from build123d import *

# Parameters (mm, degrees)
SKETCH_1_W          = 35
SKETCH_1_H          = 3
EXTRUDE_1_DEPTH     = 25
EXTRUDE_1_2_DEPTH   = 25
SKETCH_2_W          = 35
SKETCH_2_H          = 9.3
EXTRUDE_2_DEPTH     = 70
SKETCH_3_R          = 1.5
CUT_EXTRUDE_1_DEPTH = 10


with BuildPart() as part:
    # Sketch 1 → Extrude 1 (new body)
    with BuildSketch(Plane.XY):
        with Locations((17.5, 1.5)):
            Rectangle(SKETCH_1_W, SKETCH_1_H)
    extrude(amount=EXTRUDE_1_DEPTH)



with BuildPart() as body_2:
    # Sketch 1 → Extrude 1 2 (new body)
    with BuildSketch(Plane.XY):
        with Locations((17.5, -4.8)):
            Rectangle(SKETCH_1_W, SKETCH_1_H)
    extrude(amount=EXTRUDE_1_2_DEPTH)


with BuildPart() as part_1:
    add(part.part)

    add(body_2.part)  # Extrude 2 merges body 2
    # Sketch 2 → Extrude 2 (add)
    with BuildSketch(Plane(origin=(0, 0, 0), x_dir=(-1, 0, 0), z_dir=(0, 0, -1))):
        with Locations((-17.5, -1.65)):
            Rectangle(SKETCH_2_W, SKETCH_2_H)
    extrude(amount=EXTRUDE_2_DEPTH)

    # Sketch 3 → Cut-Extrude 1 (cut)
    with BuildSketch(Plane(origin=(0, 3, 0), x_dir=(1, 0, 0), z_dir=(0, 1, 0))):
        with Locations(Location((7.5, -20.5, 0), (0, 0, 270))):
            Circle(SKETCH_3_R)
        with Locations(Location((17.5, -20.5, 0), (0, 0, 270))):
            Circle(SKETCH_3_R)
        with Locations(Location((27.5, -20.5, 0), (0, 0, 270))):
            Circle(SKETCH_3_R)
    extrude(amount=-CUT_EXTRUDE_1_DEPTH, mode=Mode.SUBTRACT)


solid = part_1.part
Source: CAD feature listing. Evaluate the final solid. Frame: model axes, mm. A direction names the side the tool comes from. Round coordinates to 2 decimals unless told otherwise and drop trailing zeros. Loops run counter-clockwise (first coordinate to the right, second up) from the corner with the lowest first, then second, coordinate; pieces in that order, holes last. Notation, with made-up numbers: (78, 42.5) - (134, 42.5) arc R21 ccw to (134, 47.5) - close; hole circle Ø5 at (80.25, -1). An arc over 180 degrees is marked (long way). Write item = value, one per line. Start each with the question number.
(1) Section query D-D, the plane y = -1.25. Output: boundary loops of the cut face in (x, z), plus the area to 3 significant figures.
(2) Section query C-C, the plane x = 32. Output: boundary loops of the cut face in (y, z).
(3) Section query A-A, the plane z = 20.5. State how many separate pieces and enclosed holes the cut face has, plus the area to 3 significant figures.
(4) Ray query, line 1 along X through (y, z) = (1.7, 20.5); line 2 along Y through (x, z) = (17.5, 5.5); line 3 along Z through (x, y) = (6.5, -2). Return the intervals inside material, ascending. Write a range as from..to.
(5) Pin query (flat end, axial travel): pin 1 (1 mm diameter, centred on x = 13, y = -2, fed in from +Z). Return the tip coordinate at first contact, or that it passes through.
(6) Pull-direction query (X, two-part tool) for faces 3 (the face through (18.51, 1.52, 19.39)), 4 (the face through (6.6, 1.5, 19.3)), 5 (the face through (17, 0, 12)), 6 (the face through (35, -2, -22)); classes: +X half, -X half, draft (parallel to the pull), parting line (faces both ways), or undercut.
(7) Set-up query: faces 1 (the face through (18, -6.3, -22)), 2 (the face through (18, -2, 0)). Return all of +Z, -Z, +X, -X, +Y, -Y with unobstructed straight access to the full face (end or side cutting, diameter ignored); none if empty.
(8) Section query B-B, the plane x = 17.5. Output: boundary loops of the cut face in (y, z).
Conclusion:
q1.outline = (0, -70) - (35, -70) - (35, 0) - (0, 0) - close
q1.area = 2,450 mm2
q2.outline = (-6.3, -70) - (3, -70) - (3, 25) - (0, 25) - (0, 0) - (-3.3, 0) - (-3.3, 25) - (-6.3, 25) - close
q3.separate_pieces = 8
q3.enclosed_holes = 0
q3.area = 156 mm2
q4.line_1 = 0..6, 9..16, 19..26, 29..35
q4.line_2 = -6.3..-3.3, 0..3
q4.line_3 = -70..0
q5.pin_1 = 0
q6.face_3 = undercut
q6.face_4 = undercut
q6.face_5 = draft
q6.face_6 = +X half
q7.face_1 = +Z, -Z, +X, -X, -Y
q7.face_2 = +Z, +X, -X
q8.outline = (-6.3, -70) - (3, -70) - (3, 19) - (0, 19) - (0, 0) - (-3.3, 0) - (-3.3, 19) - (-6.3, 19) - close; (-6.3, 22) - (-3.3, 22) - (-3.3, 25) - (-6.3, 25) - close; (0, 22) - (3, 22) - (3, 25) - (0, 25) - close
